```python
from build123d import *

# Parameters (mm, degrees)
SKETCH1_R           = 19.5
SKETCH1_R_2         = 2.1
SKETCH1_R_3         = 2
SKETCH1_R_4         = 2.5
SKETCH1_R_5         = 9.5
SKETCH1_R_6         = 1.25
SKETCH1_R_7         = 11
BOSS_EXTRUDE1_DEPTH = 5
SKETCH15_R          = 2
CUT_EXTRUDE14_DEPTH = 10
SKETCH18_R          = 2.5
CUT_EXTRUDE15_DEPTH = 483.844656179
FILLET2_R           = 40
FILLET3_R           = 40
SKETCH21_W          = 20
SKETCH21_H          = 8
BOSS_EXTRUDE3_DEPTH = 5
SKETCH20_R          = 4
CUT_EXTRUDE17_DEPTH = 279.07373123
FILLET4_R           = 4
FILLET5_R           = 3


with BuildPart() as part:
    # Sketch1 → Boss-Extrude1 (new body)
    with BuildSketch(Plane(origin=(0, 0, 0), x_dir=(1, 0, 0), z_dir=(0, 1, 0))):
        with BuildLine():
            Line((0, 85), (0, 0))
            Line((0, 0), (220, 0))
            Line((220, 0), (220, 46))
            Line((220, 46), (210, 70))
            Line((210, 70), (210, 130))
            ThreePointArc((210, 130), (170, 170), (130, 130))
            Line((130, 130), (130, 110))
            ThreePointArc((130, 110), (127.071067812, 102.928932188), (120, 100))
            Line((120, 100), (15, 100))
            ThreePointArc((15, 100), (4.393398282, 95.606601718), (0, 85))
        make_face()
        with Locations(Location((41.3, 52.378949376, 0), (0, 0, 270))):
            Circle(SKETCH1_R, mode=Mode.SUBTRACT)
        with Locations(Location((95.75, 52.378949376, 0), (0, 0, 270))):
            Circle(SKETCH1_R_2, mode=Mode.SUBTRACT)
        with BuildLine():
            ThreePointArc((74.29628188, 89.247443853), (77.033008956, 80.00277522), (77.543356768, 70.375048681))
            ThreePointArc((77.543356768, 70.375048681), (73.293969575, 66.641055044), (69.559975938, 70.890442238))
            ThreePointArc((69.559975938, 70.890442238), (69.148853816, 78.646273201), (66.944221964, 86.093523278))
            ThreePointArc((66.944221964, 86.093523278), (69.043291634, 91.346513523), (74.29628188, 89.247443853))
        make_face(mode=Mode.SUBTRACT)
        with Locations(Location((115.75, 32.378949376, 0), (0, 0, 270))):
            Circle(SKETCH1_R_2, mode=Mode.SUBTRACT)
        with Locations(Location((148.636752457, 37.233182234, 0), (0, 0, 270))):
            Circle(SKETCH1_R_3, mode=Mode.SUBTRACT)
        with Locations(Location((185, 22, 0), (0, 0, 270))):
            Circle(SKETCH1_R_4, mode=Mode.SUBTRACT)
        with Locations(Location((195, 30, 0), (0, 0, 270))):
            Circle(SKETCH1_R_3, mode=Mode.SUBTRACT)
        with Locations(Location((115.75, 52.378949376, 0), (0, 0, 270))):
            Circle(SKETCH1_R_5, mode=Mode.SUBTRACT)
        with Locations(Location((135.75, 52.378949376, 0), (0, 0, 270))):
            Circle(SKETCH1_R_2, mode=Mode.SUBTRACT)
        with Locations(Location((115.75, 72.378949376, 0), (0, 0, 270))):
            Circle(SKETCH1_R_2, mode=Mode.SUBTRACT)
        with Locations(Location((127.63485968, 84.474011316, 0), (0, 0, 270))):
            Circle(SKETCH1_R_6, mode=Mode.SUBTRACT)
        with BuildLine():
            ThreePointArc((164.775508993, 80.152802956), (168.201540304, 66.369956658), (163.138904602, 53.100658923))
            ThreePointArc((163.138904602, 53.100658923), (157.520629535, 52.441124786), (156.861095398, 58.059399852))
            ThreePointArc((156.861095398, 58.059399852), (160.216140339, 66.853058501), (157.94568485, 75.987049461))
            ThreePointArc((157.94568485, 75.987049461), (159.277720174, 81.48483828), (164.775508993, 80.152802956))
        make_face(mode=Mode.SUBTRACT)
        with Locations(Location((140, 85, 0), (0, 0, 270))):
            Circle(SKETCH1_R_4, mode=Mode.SUBTRACT)
        with Locations(Location((192.472842847, 57.698975127, 0), (0, 0, 270))):
            Circle(SKETCH1_R_6, mode=Mode.SUBTRACT)
        with Locations(Location((205.365861758, 46, 0), (0, 0, 270))):
            Circle(SKETCH1_R_3, mode=Mode.SUBTRACT)
        with Locations(Location((175.551473485, 74.952011351, 0), (0, 0, 270))):
            Circle(SKETCH1_R_6, mode=Mode.SUBTRACT)
        with Locations(Location((200, 70, 0), (0, 0, 270))):
            Circle(SKETCH1_R_4, mode=Mode.SUBTRACT)
        with Locations(Location((9.83558927, 89.725342507, 0), (0, 0, 270))):
            Circle(SKETCH1_R_4, mode=Mode.SUBTRACT)
        with Locations(Location((84.83558927, 89.725342507, 0), (0, 0, 270))):
            Circle(SKETCH1_R_4, mode=Mode.SUBTRACT)
        with Locations(Location((105.63485968, 94.474011316, 0), (0, 0, 270))):
            Circle(SKETCH1_R_6, mode=Mode.SUBTRACT)
        with Locations(Location((170, 105, 0), (0, 0, 270))):
            Circle(SKETCH1_R_2, mode=Mode.SUBTRACT)
        with Locations(Location((145, 130, 0), (0, 0, 270))):
            Circle(SKETCH1_R_2, mode=Mode.SUBTRACT)
        with Locations(Location((170, 130, 0), (0, 0, 270))):
            Circle(SKETCH1_R_7, mode=Mode.SUBTRACT)
        with Locations(Location((195, 130, 0), (0, 0, 270))):
            Circle(SKETCH1_R_2, mode=Mode.SUBTRACT)
        with Locations(Location((170, 155, 0), (0, 0, 270))):
            Circle(SKETCH1_R_2, mode=Mode.SUBTRACT)
    extrude(amount=BOSS_EXTRUDE1_DEPTH)

    # Sketch15 → Cut-Extrude14 (cut)
    with BuildSketch(Plane(origin=(0, 5, 0), x_dir=(1, 0, 0), z_dir=(0, 1, 0))):
        with Locations(Location((41.3, 85.711963041, 0), (0, 0, 270))):
            Circle(SKETCH15_R)
        with Locations(Location((74.633013665, 52.378949376, 0), (0, 0, 270))):
            Circle(SKETCH15_R)
        with Locations(Location((41.3, 19.045935711, 0), (0, 0, 270))):
            Circle(SKETCH15_R)
        with Locations(Location((7.966986335, 52.378949376, 0), (0, 0, 270))):
            Circle(SKETCH15_R)
    extrude(amount=-CUT_EXTRUDE14_DEPTH, mode=Mode.SUBTRACT)

    # Sketch18 → Cut-Extrude15 (cut, through all)
    with BuildSketch(Plane(origin=(300.638016231, 0, 207.797227621), x_dir=(-1, 0, 0), z_dir=(0, -1, 0))):
        with Locations(Location((292.118016257, 224.797227621, 0), (0, 0, 90))):
            Circle(SKETCH18_R)
        with Locations(Location((224.458016257, 224.797227621, 0), (0, 0, 90))):
            Circle(SKETCH18_R)
        with Locations(Location((156.798016257, 224.797227621, 0), (0, 0, 90))):
            Circle(SKETCH18_R)
        with Locations(Location((89.138016257, 224.797227621, 0), (0, 0, 90))):
            Circle(SKETCH18_R)
        with BuildLine():
            Line((293.118016257, 229.397227621), (291.118016257, 229.397227621))
            ThreePointArc((291.118016257, 229.397227621), (289.718016257, 230.797227621), (291.118016257, 232.197227621))
            Line((291.118016257, 232.197227621), (293.118016257, 232.197227621))
            ThreePointArc((293.118016257, 232.197227621), (294.518016257, 230.797227621), (293.118016257, 229.397227621))
        make_face()
        with BuildLine():
            Line((293.118016257, 213.397227621), (291.118016257, 213.397227621))
            ThreePointArc((291.118016257, 213.397227621), (289.718016257, 214.797227621), (291.118016257, 216.197227621))
            Line((291.118016257, 216.197227621), (293.118016257, 216.197227621))
            ThreePointArc((293.118016257, 216.197227621), (294.518016257, 214.797227621), (293.118016257, 213.397227621))
        make_face()
        with BuildLine():
            Line((225.458016257, 229.397227621), (223.458016257, 229.397227621))
            ThreePointArc((223.458016257, 229.397227621), (222.058016257, 230.797227621), (223.458016257, 232.197227621))
            Line((223.458016257, 232.197227621), (225.458016257, 232.197227621))
            ThreePointArc((225.458016257, 232.197227621), (226.858016257, 230.797227621), (225.458016257, 229.397227621))
        make_face()
        with BuildLine():
            Line((225.458016257, 213.397227621), (223.458016257, 213.397227621))
            ThreePointArc((223.458016257, 213.397227621), (222.058016257, 214.797227621), (223.458016257, 216.197227621))
            Line((223.458016257, 216.197227621), (225.458016257, 216.197227621))
            ThreePointArc((225.458016257, 216.197227621), (226.858016257, 214.797227621), (225.458016257, 213.397227621))
        make_face()
        with BuildLine():
            Line((157.798016257, 229.397227621), (155.798016257, 229.397227621))
            ThreePointArc((155.798016257, 229.397227621), (154.398016257, 230.797227621), (155.798016257, 232.197227621))
            Line((155.798016257, 232.197227621), (157.798016257, 232.197227621))
            ThreePointArc((157.798016257, 232.197227621), (159.198016257, 230.797227621), (157.798016257, 229.397227621))
        make_face()
        with BuildLine():
            Line((157.798016257, 213.397227621), (155.798016257, 213.397227621))
            ThreePointArc((155.798016257, 213.397227621), (154.398016257, 214.797227621), (155.798016257, 216.197227621))
            Line((155.798016257, 216.197227621), (157.798016257, 216.197227621))
            ThreePointArc((157.798016257, 216.197227621), (159.198016257, 214.797227621), (157.798016257, 213.397227621))
        make_face()
        with BuildLine():
            Line((90.138016257, 229.697227621), (88.138016257, 229.697227621))
            ThreePointArc((88.138016257, 229.697227621), (86.738016257, 231.097227621), (88.138016257, 232.497227621))
            Line((88.138016257, 232.497227621), (90.138016257, 232.497227621))
            ThreePointArc((90.138016257, 232.497227621), (91.538016257, 231.097227621), (90.138016257, 229.697227621))
        make_face()
        with BuildLine():
            Line((90.138016257, 213.697227621), (88.138016257, 213.697227621))
            ThreePointArc((88.138016257, 213.697227621), (86.738016257, 215.097227621), (88.138016257, 216.497227621))
            Line((88.138016257, 216.497227621), (90.138016257, 216.497227621))
            ThreePointArc((90.138016257, 216.497227621), (91.538016257, 215.097227621), (90.138016257, 213.697227621))
        make_face()
    extrude(amount=-CUT_EXTRUDE15_DEPTH, mode=Mode.SUBTRACT)

    # Fillet2
    fillet2_edges = [part.edges().sort_by_distance(p)[0] for p in [
        (210, 2.5, -70),
    ]]
    fillet(fillet2_edges, radius=FILLET2_R)

    # Fillet3
    fillet3_edges = [part.edges().sort_by_distance(p)[0] for p in [
        (220, 2.5, -46),
    ]]
    fillet(fillet3_edges, radius=FILLET3_R)

    # Sketch21 → Boss-Extrude3 (add)
    with BuildSketch(Plane.XZ):
        with Locations((30, -104)):
            Rectangle(SKETCH21_W, SKETCH21_H)
    extrude(amount=-BOSS_EXTRUDE3_DEPTH)

    # Sketch20 → Cut-Extrude17 (cut, through all)
    with BuildSketch(Plane(origin=(0, 0, 0), x_dir=(-1, 0, 0), z_dir=(0, -1, 0))):
        with Locations(Location((-31, 99, 0), (0, 0, 90))):
            Circle(SKETCH20_R)
    extrude(amount=-CUT_EXTRUDE17_DEPTH, mode=Mode.SUBTRACT)

    # Fillet4
    fillet4_edges = [part.edges().sort_by_distance(p)[0] for p in [
        (40, 2.5, -100),
        (20, 2.5, -100),
    ]]
    fillet(fillet4_edges, radius=FILLET4_R)
    fillet4_2_edges = [part.edges().sort_by_distance(p)[0] for p in [
        (40, 2.5, -108),
        (20, 2.5, -108),
    ]]
    fillet(fillet4_2_edges, radius=FILLET4_R - 0.0001)  # a hair under: the kernel refuses the full size

    # Fillet5
    fillet5_edges = [part.edges().sort_by_distance(p)[0] for p in [
        (220, 2.5, 0),
        (0, 2.5, 0),
    ]]
    fillet(fillet5_edges, radius=FILLET5_R)


solid = part.part
```
Check sheet for the modelled part. Datum: model origin and axes. Units: mm. A direction names the side the tool comes from. Give positions to 0.01 mm unless a question says otherwise; leave off trailing zeros. Order: outer loops, then holes, each group sorted by start corner. A loop starts at its lowest first (then second) coordinate and runs counter-clockwise, first axis right, second up. Notation, with made-up numbers: (85.25, 30) -> (92.25, 30) arc R11 ccw to (92.25, 50) -> close; hole circle Ø3 at (48.5, -11.5). An arc over 180 degrees is marked (long way). Return JSON: item names as keys, results as strings.
1. Cross-section at C-C, the plane z = -115. Record the cut outline in (x, y), plus the area to 3 significant figures.
From the geometry:
{"outline": "(130, 0) -> (210, 0) -> (210, 5) -> (130, 5) -> close", "area": "400 mm^2"}
2. Set-up check for faces 5 (the cylindrical face through (77.01, 2.46, -80.14)), 6 (the flat face through (30, 2, -108)), 7 (the flat face through (83, 2, -100)): record each of +Z, -Z, +X, -X, +Y, -Y from which the full face is reachable in a straight line by a thin tool's end or side.
From the geometry:
{"face 5": "+Y, -Y", "face 6": "-Z, -X, +Y, -Y", "face 7": "-Z, +Y, -Y"}
3. Mould release check, pull along X, two halves, no side actions. Record for faces 1 (the cylindrical face through (170.88, 2.46, -169.99)), 2 (the cylindrical face through (196.77, 2.46, -128.87)), 3 (the flat face through (210, 2, -104)), 4 (the flat face through (133, 0, -67)): +X half, -X half, draft (parallel to the pull), parting line (faces both ways), or undercut.
From the geometry:
{"face 1": "parting line", "face 2": "undercut", "face 3": "+X half", "face 4": "draft"}
4. Go/stop test with flat-tipped pins: P1, Ø5, axis at x = 151, z = -73, coming from the -Y side; P2, Ø1.5, axis at y = 2, z = -116.5, coming from the -X side; P3, Ø2, axis at x = 105.63, z = -94.47, coming from the +Y side; P4, Ø3, axis at y = 2, z = -125.5, coming from the +X side. Record where each tip stops, or that it passes through.
From the geometry:
{"P1": "y = 0", "P2": "x = 130", "P3": "through", "P4": "x = 210"}
5. Cross-section at B-B, the plane y = 4.1. Count the separate pieces of the cut face and the enclosed holes in it, plus the area to 3 significant figures.
From the geometry:
{"separate pieces": "1", "enclosed holes": "42", "area": "23,800 mm^2"}
6. Material ranges on probe 1 along Z at (x, y) = (85, 2.05); probe 2 along X at (y, z) = (1.5, -85); probe 3 along X at (y, z) = (2.8, -68), recorded low to high. Write a range as [from, to].
From the geometry:
{"probe 1": "[-100, -92.22], [-87.23, 0]", "probe 2": "[0, 39.43], [43.17, 67.39], [75.85, 126.5], [128.77, 137.5], [142.5, 210]", "probe 3": "[0, 29.63], [52.97, 70.54], [76.56, 160.24], [168.24, 198.5], [201.5, 211.27]"}
7. Cross-section at A-A, the plane z = -134.5. Record the cut outline in (x, y), plus the area to 3 significant figures.
From the geometry:
{"outline": "(130.25, 0) -> (159.96, 0) -> (159.96, 5) -> (130.25, 5) -> close; (180.04, 0) -> (209.75, 0) -> (209.75, 5) -> (180.04, 5) -> close", "area": "297 mm^2"}
